Autodesk Inventor part; units mm, degrees
ref_plane "YZ Plane" through (0, 0, 0) normal (1, 0, 0) x (0, 1, 0)
ref_plane "XZ Plane" through (0, 0, 0) normal (0, 1, 0) x (-1, 0, 0)
ref_plane "XY Plane" through (0, 0, 0) normal (0, 0, 1) x (1, 0, 0)
sketch "Sketch1" plane through (0, 0, 0) normal (0, 1, 0) x (-1, 0, 0)
  line L0 (0, 0) -> (-20, 0)
  line L1 (-20, 0) -> (-20, -100)
  line L2 (-20, -100) -> (0, -100)
  line L3 (0, -100) -> (0, 0)
  line L4 (-10, 0) -> (-10, -6)
  line L5 (-10, -6) -> (60, -6) construction
  line L6 (-10, -6) -> (-10, -26) construction
  line L7 (-13, -6) -> (-13, -26)
  line L8 (-7, -26) -> (-7, -6)
  arc A0 (-7, -6) -> (-13, -6) centre (-10, -6) ccw
  arc A1 (-13, -26) -> (-7, -26) centre (-10, -26) ccw
  line L9 (-10, -100) -> (-10, -94)
  line L10 (-10, -94) -> (-10, -74) construction
  line L11 (-7, -94) -> (-7, -74)
  line L12 (-13, -74) -> (-13, -94)
  arc A2 (-13, -94) -> (-7, -94) centre (-10, -94) ccw
  arc A3 (-7, -74) -> (-13, -74) centre (-10, -74) ccw
  point P0 (-10, -16)
  point P1 (-10, -84)
  dimension "d0" = 20
  dimension "d1" = 100
  dimension "d2" = 6
  dimension "d9" = 20
  dimension "d10" = 6
  dimension "d11" = 6
  dimension "d12" = 20
  dimension "d13" = 6
extrude "Extrusion1" add sketch "Sketch1" along normal blind 6
fillet "Fillet1" radius 5 4 edges at (20, 3, 0) (0, 3, 0) (20, 3, -100) (0, 3, -100)
properties part number "Carriage_Horizontal_Spacer"
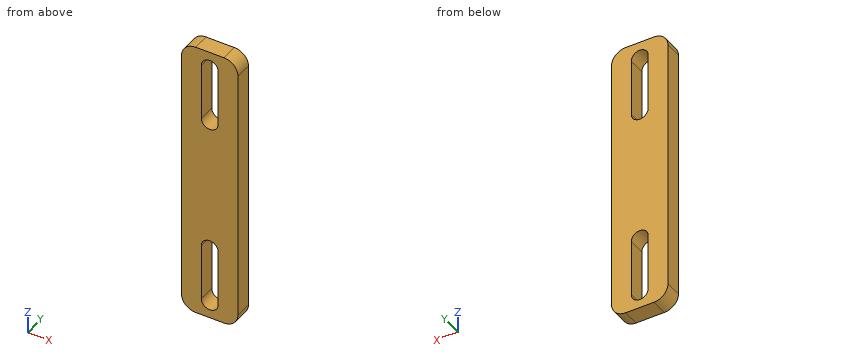
Check sheet for the modelled part. Datum: model origin and axes. Units: mm. Give positions to 0.01 mm unless a question says otherwise; leave off trailing zeros. Loops run counter-clockwise (first coordinate to the right, second up) from the corner with the lowest first, then second, coordinate; pieces in that order, holes last. Notation, with made-up numbers: (47, 76) - (100, 76) arc R11 cw to (100, 83) - close; hole circle Ø9 at (-17, 9). An arc over 180 degrees is marked (long way). One line per question, with ' | ' between items. Start each with the question number.
1. Gauge pin test, flat ends, axial feed: pin 1 Ø3 at (y, z) = (2.5, -83) entering from -X; pin 2 Ø3 at (x, y) = (2.5, 1) entering from +Z. Record the tip position at first contact, or that the pin passes through.
2. Cross-section at C-C, the plane y = 0.9. Enter the section's corners in (x, z).
3. Material ranges on line 1 along X through (y, z) = (3.2, -15.5); line 2 along Z through (x, y) = (12.25, 3.95); line 3 along Z through (x, y) = (8, 3.6), recorded low to high. Write a range as [from, to].
4. Cross-section at B-B, the plane z = -23. Enter the section's corners in (x, y).
5. Cross-section at A-A, the plane x = 10. Enter the section's corners in (y, z), plus the area to 3 significant figures.
Check result:
1) pin 1: stops at x = 0 | pin 2: stops at z = -0.1
2) outline: (0, -95) arc R5 ccw to (5, -100) - (15, -100) arc R5 ccw to (20, -95) - (20, -5) arc R5 ccw to (15, 0) - (5, 0) arc R5 ccw to (0, -5) - close; hole (7, -94) arc R3 ccw to (13, -94) - (13, -74) arc R3 ccw to (7, -74) - close; hole (7, -26) arc R3 ccw to (13, -26) - (13, -6) arc R3 ccw to (7, -6) - close
3) line 1: x = [0, 7], [13, 20] | line 2: z = [-100, -95.98], [-72.02, -27.98], [-4.02, 0] | line 3: z = [-100, -96.24], [-71.76, -28.24], [-3.76, 0]
4) outline: (0, 0) - (7, 0) - (7, 6) - (0, 6) - close; (13, 0) - (20, 0) - (20, 6) - (13, 6) - close
5) outline: (0, -100) - (6, -100) - (6, -97) - (0, -97) - close; (0, -71) - (6, -71) - (6, -29) - (0, -29) - close; (0, -3) - (6, -3) - (6, 0) - (0, 0) - close | area: 288 mm2
